Source: CAD feature listing. Evaluate the final solid. Frame: model axes, mm. A direction names the side the tool comes from. Round coordinates to 2 decimals unless told otherwise and drop trailing zeros. Return JSON: item names as keys, results as strings. Group by question number.
1) Ray query, line 1 (Z direction, x = 0, y = 221); line 2 (X direction, y = 334.5, z = 6). Return the intervals inside material, ascending. Write a range as from..to.
2) Contact query for flat-ended pins moving along their axis: P1, Ø1.7, axis at x = 1, y = 258, coming from the +Z side; P2, Ø6, axis at x = 1, y = 101.5, coming from the -Z side. Output: stop coordinate, or through.
3) Access query for faces 1 (the flat face through (0.1, 350, -2.4)), 2 (the flat face through (-3.9, 173, 0)). Directions: +Z, -Z, +X, -X, +Y, -Y. A direction counts if a zero-diameter tool reaches every point of the face in a straight line with its end or side. Return the directions, or none.
4) Mould query, pull axis Z, two halves, no side actions, for faces 3 (the flat face through (0, 173, 3.9)), 4 (the flat face through (3.9, 173, 0)), 5 (the flat face through (0, 173, -3.9)). Classes: pulls with the +Z half, pulls with the -Z half, needs draft (parallel to the pull), parting line crosses it, or undercut.
```python
from build123d import *

# Parameters (mm, degrees)
SKETCH_1_R      = 2.1
EXTRUDE_1_DEPTH = 350


with BuildPart() as part:
    # 草图1 → 凸台-拉伸1 (new body)
    with BuildSketch(Plane(origin=(0, 0, 0), x_dir=(1, 0, 0), z_dir=(0, 1, 0))):
        Polygon((-10, 10), (-4.9, 10), (-3.1, 8.2), (-5.5, 8.2), (-5.5, 6.560660172), (-2.839339828, 3.9), (0, 3.9), (2.839339828, 3.9), (5.5, 6.560660172), (5.5, 8.2), (3.1, 8.2), (4.9, 10), (10, 10), (10, 4.9), (8.2, 3.1), (8.2, 5.5), (6.560660172, 5.5), (3.9, 2.839339828), (3.9, -2.839339828), (6.560660172, -5.5), (8.2, -5.5), (8.2, -3.1), (10, -4.9), (10, -10), (4.9, -10), (3.1, -8.2), (5.5, -8.2), (5.5, -6.560660172), (2.839339828, -3.9), (0, -3.9), (-2.839339828, -3.9), (-5.5, -6.560660172), (-5.5, -8.2), (-3.1, -8.2), (-4.9, -10), (-10, -10), (-10, -4.9), (-8.2, -3.1), (-8.2, -5.5), (-6.560660172, -5.5), (-3.9, -2.839339828), (-3.9, 2.839339828), (-6.560660172, 5.5), (-8.2, 5.5), (-8.2, 3.1), (-10, 4.9), align=None)
        Circle(SKETCH_1_R, mode=Mode.SUBTRACT)
    extrude(amount=EXTRUDE_1_DEPTH)


solid = part.part
```
Geometry check:
{
 "1": {"line 1": "-3.9..-2.1, 2.1..3.9", "line 2": "-10..-4.94, 4.94..10"},
 "2": {"P1": "z = 3.9", "P2": "z = -9.1"},
 "3": {"face 1": "+Z, -Z, +X, -X, +Y", "face 2": "-X, +Y, -Y"},
 "4": {"face 3": "pulls with the +Z half", "face 4": "undercut", "face 5": "pulls with the -Z half"}
}
